Autodesk Fusion 360 part; units mm, degrees
sketch "Sketch1" plane through (0, 0, 0) normal (0, 1, 0) x (1, 0, 0)
  line L0 (17, -4) -> (-17, -4)
  line L1 (-17, -4) -> (-17, 4)
  line L2 (-17, 4) -> (17, 4)
  line L3 (17, 4) -> (17, -4)
  line L4 (17, -4) -> (-17, 4) construction
  line L5 (-17, -4) -> (17, 4) construction
  circle A0 centre (-13, 0) radius 1.6
  circle A1 centre (13, 0) radius 1.6
  line L6 (-13, 0) -> (0, 0) construction
  line L7 (0, 0) -> (13, 0) construction
  dimension "d1" = 26
  dimension "d2" = 3.2
  dimension "d3" = 34
  dimension "d4" = 8
extrude "Extrude1" add sketch "Sketch1" along normal blind 13.8
sketch "Sketch3" plane through (0, 0, 4) normal (0, 0, 1) x (-1, 0, 0)
  line L0 (17, 0) -> (-17, 0)
  line L1 (-17, 0) -> (-17, -13.8)
  line L2 (-17, -13.8) -> (17, -13.8)
  line L3 (17, -13.8) -> (17, 0)
  line L4 (0, 0) -> (0, -13.8) construction
  line L5 (0, -11.5) -> (-7.5, -11.5) construction
  line L6 (0, -11.5) -> (7.5, -11.5) construction
  circle A0 centre (7.5, -11.5) radius 0.8
  circle A1 centre (-7.5, -11.5) radius 0.8
  dimension "d7" = 15
  dimension "d8" = 1.6
  dimension "d9" = 2.3
extrude "Extrude2" cut sketch "Sketch3" against normal through all contours A0 | A1
sketch "Sketch5" plane through (0, 13.8, 0) normal (0, 1, 0) x (-1, 0, 0)
  circle A0 centre (-13, 0) radius 1.6
  circle A1 centre (13, 0) radius 1.6
  line L0 (-17, -4) -> (17, -4)
  line L1 (17, -4) -> (17, 4)
  line L2 (17, 4) -> (-17, 4)
  line L3 (-17, 4) -> (-17, -4)
  circle A2 centre (-13, 0) radius 2.95
  circle A3 centre (13, 0) radius 2.95
  dimension "d11" = 5.9
extrude "Extrude3" add sketch "Sketch5" along normal blind 1.2 contours A2 | A3
fillet "Fillet1" radius 0.4 2 edges at (15.7504, 15, -1.0668) (-10.2496, 15, -1.0668)
extrude "Extrude4" cut 1 faces at (4.1385, 0, 3.1631) along direction (0, 1, 0) blind 10
sketch "Sketch7" plane through (0, 10, 0) normal (0, -1, 0) x (1, 0, 0)
  circle A0 centre (13, 0) radius 1.6
  circle A1 centre (-13, 0) radius 1.6
  line L0 (-17, -4) -> (17, -4)
  line L1 (17, -4) -> (17, 4)
  line L2 (17, 4) -> (-17, 4)
  line L3 (-17, 4) -> (-17, -4)
  circle A2 centre (-13, 0) radius 3
  circle A3 centre (13, 0) radius 3
  line L4 (-10.3, 4) -> (10.3, 4)
  line L5 (10.3, 4) -> (10.3, 2)
  line L6 (10.3, 2) -> (-10.3, 2)
  line L7 (-10.3, 2) -> (-10.3, 4)
  line L8 (-8.3, 4) -> (-6.7, 4)
  line L9 (6.7, 4) -> (8.3, 4)
  line L10 (-9.3, 2) -> (9.3, 2)
  line L11 (9.3, 2) -> (9.3, -4)
  line L12 (9.3, -4) -> (-9.3, -4)
  line L13 (-9.3, -4) -> (-9.3, 2)
  dimension "d20" = 6
  dimension "d21" = 6
  dimension "d22" = 2
  dimension "d23" = 2
  dimension "d24" = 2
  dimension "d25" = 1
  dimension "d26" = 1
extrude "Extrude5" add sketch "Sketch7" along normal blind 1 contours L0 L6 L10 L11 L12 L13 | L2 L4 L5 L6 L7 L8 L9 L10
sketch "Sketch8" plane through (0, 9, 0) normal (0, -1, 0) x (1, 0, 0)
  line L0 (-9.3, -4) -> (9.3, -4)
  line L1 (9.3, -4) -> (9.3, 2)
  line L2 (9.3, 2) -> (10.3, 2)
  line L3 (10.3, 2) -> (10.3, 4)
  line L4 (10.3, 4) -> (-10.3, 4)
  line L5 (-10.3, 4) -> (-10.3, 2)
  line L6 (-10.3, 2) -> (-9.3, 2)
  line L7 (-9.3, 2) -> (-9.3, -4)
  line L8 (-10.3, 4) -> (10.3, 4)
  line L9 (10.3, 4) -> (10.3, 2)
  line L10 (10.3, 2) -> (-10.3, 2)
  line L11 (-10.3, 2) -> (-10.3, 4)
extrude "Extrude6" add sketch "Sketch8" along normal blind 6 contours L2 L3 L4 L5 L6 L8 L9 L10 L11
fillet "Fillet3" radius 2 1 edges at (0, 9, 2)
fillet "Fillet4" radius 3 2 edges at (17, 11.9, -4) (-17, 11.9, -4)
chamfer "Chamfer1" distance 2 angle 45 2 edges at (-17, 11.9, 4) (17, 11.9, 4)
sketch "Sketch9" plane through (-17, 0, 0) normal (-1, 0, 0) x (0, -1, 0)
  line L0 (-10, 2) -> (-13.8, 2)
  line L1 (-13.8, 2) -> (-13.8, -1)
  line L2 (-13.8, -1) -> (-10, -1)
  line L3 (-10, -1) -> (-10, 2)
  line L4 (-13.8, -2.95) -> (-13.8, 2.95)
  line L5 (-14.6, 2.95) -> (-14.6, -2.95) construction
  line L6 (-15, -2.55) -> (-15, 2.55)
  line L7 (-13.8, 2.95) -> (-15, 1.75)
  line L8 (-13.8, 2.95) -> (-15, 2.95)
  line L9 (-15, 1.75) -> (-15, 2.95)
  dimension "d36" = 45
extrude "Extrude7" cut sketch "Sketch9" against normal through all contours L6 L7 L8 L9
chamfer "Chamfer2" distance 0.6 angle 45 2 edges at (-10.3, 6.5, 2) (10.3, 6.5, 2)
sketch "Sketch10" plane through (0, 13.8, 0) normal (0, 1, 0) x (-1, 0, 0)
  line L0 (-15, 4) -> (-17, 2)
  line L1 (-17, 2) -> (-17, -1)
  arc A0 (-17, -1) -> (-14, -4) centre (-14, -1) ccw
  line L2 (-14, -4) -> (14, -4)
  arc A1 (14, -4) -> (17, -1) centre (14, -1) ccw
  line L3 (17, -1) -> (17, 2)
  line L4 (17, 2) -> (15, 4)
  line L5 (15, 4) -> (-15, 4)
  circle A2 centre (-13, 0) radius 2.95
  circle A3 centre (13, 0) radius 2.95
  line L6 (-13, 0) -> (-6.3, 0) construction
  line L7 (-6.3, 0) -> (-6.3, 3.25) construction
  circle A4 centre (-6.3, 3.25) radius 3
  dimension "d39" = 6.7
  dimension "d40" = 3.25
  dimension "d41" = 6
extrude "Extrude8" cut sketch "Sketch10" against normal blind 0.6 contours L5 A4 picked at (-5.6314, 4.4936)
CAD build for the part. Positions are in the model's coordinates, mm. A direction names the side the tool comes from. Give positions to 0.01 mm unless a question says otherwise; leave off trailing zeros. Order: outer loops, then holes, each group sorted by start corner. A loop starts at its lowest first (then second) coordinate and runs counter-clockwise, first axis right, second up. Notation, with made-up numbers: M 80.25,14 L 114.25,14 A17 ccw 114.25,34 Z; hole C 73,3.5 d9. An arc over 180 degrees is marked long. Put each result on its own line as item: value. Start each with the question number.
(1) Flat gauge pins, fed straight in: pin 1 Ø2 at (x, y) = (7.5, 11.5) entering from +Z; pin 2 Ø2 at (x, z) = (0, -2.5) entering from -Y; pin 3 Ø0.7 at (y, z) = (6, 3.5) entering from -X; pin 4 Ø1.1 at (y, z) = (6.5, 3.5) entering from +X. Where does each tip first touch, or does it go through?
(2) Drill centre lines: line 1 along Y through (x, z) = (-7.5, -1.75); line 2 along Z through (x, y) = (13, 12.95); line 3 along X through (y, z) = (13.5, -1). Where is each one in solid material? Low to high.
(3) Saw through at A-A, the plane x = 7.5. Write the cut outline in (y, z).
(4) Mould opens along Y. For faces 6 (the flat face through (10.3, 7, 3)), 7 (the cylindrical face through (8.09, 10.96, 0.06)), 8 (the cylindrical face through (-0.13, 8.4, 1.43)) say: +Y half, -Y half, draft (parallel to the pull), parting line (faces both ways), or undercut.
(5) Which spindle directions (+Z, -Z, +X, -X, +Y, -Y) get a long thin tool onto all of the face, cutting with end or side? Do faces 1 (the flat face through (-10.3, 7, 3)), 2 (the flat face through (-9.3, 9.5, -1)), 3 (the flat face through (0, 13.8, 0)), 4 (the flat face through (-13, 15, -2)), 5 (the flat face through (-13.03, 14.52, 2.23)). Say none if no direction does.
(6) Saw through at C-C, the plane x = -9. Write the cut outline in (y, z), then the cut area to 3 significant figures.
(7) Saw through at B-B, the plane y = 11.5. Write the cut outline in (x, z).
(8) Saw through at D-D, the plane y = 5.25. Write the cut outline in (x, z).
Check result:
1. pin 1: stops at z = 4
1. pin 2: stops at y = 9
1. pin 3: stops at x = -10.3
1. pin 4: stops at x = 10.3
2. line 1: y = 9 to 10.7, 12.3 to 13.8
2. line 2: z = -4 to -1.6, 1.6 to 4
2. line 3: x = -17 to -14.25, -11.75 to 11.75, 14.25 to 17
3. outline: M 3,2 L 7,2 A2 cw 9,0 L 9,-4 L 10.7,-4 L 10.7,4 L 3,4 Z; M 12.3,-4 L 13.8,-4 L 13.8,4 L 12.3,4 Z
4. face 6: draft
4. face 7: undercut
4. face 8: -Y half
5. face 1: +Z, -Z, -X, -Y
5. face 2: -Z, -X, -Y
5. face 3: +Y
5. face 4: +Z, -Z, +X, -X, +Y
5. face 5: +Z, +X, -X, +Y
6. outline: M 3,2 L 7,2 A2 cw 9,0 L 9,-4 L 13.8,-4 L 13.8,4 L 3,4 Z
6. area: 51.3 mm2
7. outline: M -17,-1 A3 ccw -14,-4 L -8.3,-4 L -8.3,4 L -15,4 L -17,2 Z; M -6.7,-4 L 6.7,-4 L 6.7,4 L -6.7,4 Z; M 8.3,-4 L 14,-4 A3 ccw 17,-1 L 17,2 L 15,4 L 8.3,4 Z; hole C -13,0 d3.2; hole C 13,0 d3.2
8. outline: M -10.3,2.6 L -9.7,2 L 9.7,2 L 10.3,2.6 L 10.3,4 L -10.3,4 Z
